```python
from build123d import *

# Parameters (mm, degrees)
SKETCH1_W             = 7.62
SKETCH1_H             = 96.52
BOSS_EXTRUDE1_DEPTH   = 7.62
SKETCH2_W             = 7.62
SKETCH2_H             = 5.08
BOSS_EXTRUDE2_DEPTH   = 7.62
SKETCH4_W             = 7.62
SKETCH4_H             = 2.54
BOSS_EXTRUDE3_DEPTH   = 8.128
BOSS_EXTRUDE4_DEPTH   = 2.54
F_6_CLEARANCE_HOLE1_D = 3.7973
CUT_EXTRUDE1_DEPTH    = 2.54
SKETCH12_W            = 7.62
SKETCH12_H            = 45.72
CUT_EXTRUDE2_DEPTH    = 2.54
FILLET2_R             = 12.7
FILLET3_R             = 2.54
SKETCH14_R            = 1.905
CUT_EXTRUDE4_DEPTH    = 99.092682214


with BuildPart() as part:
    # Sketch1 → Boss-Extrude1 (new body)
    with BuildSketch(Plane(origin=(0, 0, 0), x_dir=(0, 0, -1), z_dir=(1, 0, 0))):
        with Locations((3.81, 48.26)):
            Rectangle(SKETCH1_W, SKETCH1_H)
    extrude(amount=BOSS_EXTRUDE1_DEPTH)

    # Sketch2 → Boss-Extrude2 (add)
    with BuildSketch(Plane.ZY):
        with Locations((-3.81, 2.54)):
            Rectangle(SKETCH2_W, SKETCH2_H)
    extrude(amount=BOSS_EXTRUDE2_DEPTH)

    # Sketch4 → Boss-Extrude3 (add)
    with BuildSketch(Plane(origin=(7.62, 0, 0), x_dir=(0, 0, -1), z_dir=(1, 0, 0))):
        with Locations((3.81, 95.25)):
            Rectangle(SKETCH4_W, SKETCH4_H)
    extrude(amount=BOSS_EXTRUDE3_DEPTH)

    # Sketch5 → Boss-Extrude4 (add)
    with BuildSketch(Plane.XZ.offset(-93.98)):
        Polygon((15.748, 0), (12.974546815, -7.62), (10.434546815, -7.62), (13.208, 0), align=None)
    extrude(amount=BOSS_EXTRUDE4_DEPTH)

    # #6 Clearance Hole1 (through all)
    with Locations(Plane(origin=(0, 5.08, 0), x_dir=(1, 0, 0), z_dir=(0, 1, 0))):
        with Locations((-3.81, 3.81)):
            Hole(F_6_CLEARANCE_HOLE1_D / 2)

    # Sketch8 → Cut-Extrude1 (cut)
    with BuildSketch(Plane.XZ.offset(-93.98)):
        Polygon((15.748, -7.62), (12.974546815, -7.62), (15.748, 0), align=None)
    extrude(amount=-CUT_EXTRUDE1_DEPTH, mode=Mode.SUBTRACT)

    # Sketch12 → Cut-Extrude2 (cut)
    with BuildSketch(Plane.ZY):
        with Locations((-3.81, 27.94)):
            Rectangle(SKETCH12_W, SKETCH12_H)
    extrude(amount=-CUT_EXTRUDE2_DEPTH, mode=Mode.SUBTRACT)

    # Fillet2
    # the kernel refuses this fillet: 12.7 mm, written as the material it takes off along each edge
    with BuildSketch(Plane(origin=(0, 50.8, 19.05), x_dir=(1, 0, 0), z_dir=(0, 0, -1))) as fillet2_piece_1:
        with BuildLine():
            CenterArc((12.7, -7.62), FILLET2_R, 143.130102354, 36.869897646)
            Line((0, -7.62), (-0.254, -7.62))
            Line((-0.254, -7.62), (-0.254, 0))
            Line((-0.254, 0), (0, 0.254))
            ThreePointArc((0, 0.254), (1.27, 0.254), (2.3368, 0.1524))
            Line((2.3368, 0.1524), (2.54, 0))
        make_face()
    extrude(amount=45.72, mode=Mode.SUBTRACT)

    # Fillet3
    fillet3_edges = [part.edges().sort_by_distance(p)[0] for p in [
        (2.54, 5.08, -3.81),
        (7.62, 0, -3.81),
        (0, 96.52, -3.81),
    ]]
    fillet(fillet3_edges, radius=FILLET3_R)

    # Sketch14 → Cut-Extrude4 (cut, through all)
    with BuildSketch(Plane.XY):
        with Locations((3.81, 83.82)):
            Circle(SKETCH14_R)
        with Locations((3.81, 73.66)):
            Circle(SKETCH14_R)
    extrude(amount=-CUT_EXTRUDE4_DEPTH, mode=Mode.SUBTRACT)


solid = part.part
```
Read the model definition and answer for the solid it produces. Units are mm, in the model's axes. A direction names the side the tool comes from. Coordinates: 2 decimals unless noted, no trailing zeros. Write each loop counter-clockwise with the first axis right and the second up, starting at its lowest first coordinate (ties: lowest second). Pieces come first, ordered by that corner, then holes. Notation, with made-up numbers: (29.5, -13.5) -> (58.5, -13.5) arc R18 ccw to (58.5, 9.5) -> close; hole circle Ø9 at (-5.5, 65). An arc over 180 degrees is marked (long way). Answer as a JSON object with one key per item and string values.
Q1. Flat-ended cylindrical pins translate along their axes: pin 1 Ø2.5 at (x, y) = (3.81, 83.82) entering from -Z; pin 2 Ø4 at (x, z) = (-2.5, -4.5) entering from +Y; pin 3 Ø4 at (y, z) = (77.5, -2) entering from +X; pin 4 Ø4 at (y, z) = (34.5, -2) entering from -X. Find the tip coordinate at first contact, or state that the pin passes through.
The answers:
{"pin 1": "passes through", "pin 2": "stops at y = 5.08", "pin 3": "stops at x = 7.62", "pin 4": "stops at x = 2.54"}
Q2. The part is cut by section C-C on x = -3.81. Give the vertices of the cut face in (y, z).
The answers:
{"outline": "(0, -7.62) -> (5.08, -7.62) -> (5.08, -5.71) -> (0, -5.71) -> close; (0, -1.91) -> (5.08, -1.91) -> (5.08, 0) -> (0, 0) -> close"}
Q3. The part is cut by section B-B on x = 3.81. Give the vertices of the cut face in (y, z) (3 decimals).
The answers:
{"outline": "(0, -7.62) -> (71.755, -7.62) -> (71.755, 0) -> (0, 0) -> close; (75.565, -7.62) -> (81.915, -7.62) -> (81.915, 0) -> (75.565, 0) -> close; (85.725, -7.62) -> (96.52, -7.62) -> (96.52, 0) -> (85.725, 0) -> close"}
Q4. The part is cut by section A-A on y = 73.66. Give the vertices of the cut face in (x, z) (3 decimals).
The answers:
{"outline": "(0, -7.62) -> (1.905, -7.62) -> (1.905, 0) -> (0, 0) -> close; (5.715, -7.62) -> (7.62, -7.62) -> (7.62, 0) -> (5.715, 0) -> close"}
Q5. Determine the mould class of faces 4 (the flat face through (2.54, 30, -4)), 5 (the flat face through (-7.62, 3, -4)), 6 (the cylindrical face through (1, 96, -4)) for opening direction Y: pulls with the +Y half, pulls with the -Y half, needs draft (parallel to the pull), parting line crosses it, or undercut.
The answers:
{"face 4": "undercut", "face 5": "needs draft", "face 6": "pulls with the +Y half"}
Q6. The part is cut by section D-D on z = -3.81. Give the vertices of the cut face in (x, y) (3 decimals).
The answers:
{"outline": "(-7.62, 0) -> (-5.709, 0) -> (-5.709, 5.08) -> (-7.62, 5.08) -> close; (-1.911, 0) -> (5.08, 0) arc R2.54 ccw to (7.62, 2.54) -> (7.62, 93.98) -> (11.821, 93.98) -> (11.821, 91.44) -> (14.361, 91.44) -> (14.361, 96.52) -> (2.54, 96.52) arc R2.54 ccw to (0, 93.98) -> (0, 58.42) arc R12.7 ccw to (2.54, 50.8) -> (2.54, 7.62) arc R2.54 cw to (0, 5.08) -> (-1.911, 5.08) -> close; hole circle Ø3.81 at (3.81, 73.66); hole circle Ø3.81 at (3.81, 83.82)"}
Q7. A tool of negligible diameter and unlimited length cuts with its end or side. For faces 1 (the flat face through (0, 76, -4)), 2 (the flat face through (10, 93.98, -4)), 3 (the flat face through (13, 91.44, -4)), from which of +Z, -Z, +X, -X, +Y, -Y can it reach the whole face along a straight path? Write none if from no direction.
The answers:
{"face 1": "+Z, -Z, -X, +Y", "face 2": "+Z, -Y", "face 3": "+Z, -Z, +X, -Y"}
Q8. Consider line 1 (Y direction, x = 3.81, z = -4.25) (3 decimals); line 2 (X direction, y = 83.82, z = -3.5) (3 decimals); line 3 (Z direction, x = -3.81, y = 2.55). Determine where each line is inside the solid, lowest interval first. Write a range as [from, to].
The answers:
{"line 1": "y = [0, 71.755], [75.565, 81.915], [85.725, 96.52]", "line 2": "x = [0, 1.905], [5.715, 7.62]", "line 3": "z = [-7.62, -5.71], [-1.91, 0]"}
